from build123d import *

# Parameters (mm, degrees)
SKETCH_1_W          = 31
SKETCH_1_H          = 40
SKETCH_1_R          = 1.45
EXTRUDE_1_DEPTH     = 3
SKETCH_2_W          = 17
SKETCH_2_H          = 13
CUT_EXTRUDE_1_DEPTH = 3
FILLET_1_R          = 1.5


with BuildPart() as part:
    # 草图1 → 凸台-拉伸1 (new body)
    with BuildSketch(Plane.XY):
        with Locations((15.5, 20)):
            Rectangle(SKETCH_1_W, SKETCH_1_H)
        with Locations((4, 30)):
            Circle(SKETCH_1_R, mode=Mode.SUBTRACT)
        with Locations((4, 20)):
            Circle(SKETCH_1_R, mode=Mode.SUBTRACT)
        with Locations((4, 10)):
            Circle(SKETCH_1_R, mode=Mode.SUBTRACT)
        with Locations((27, 30)):
            Circle(SKETCH_1_R, mode=Mode.SUBTRACT)
        with Locations((27, 20)):
            Circle(SKETCH_1_R, mode=Mode.SUBTRACT)
        with Locations((27, 10)):
            Circle(SKETCH_1_R, mode=Mode.SUBTRACT)
    extrude(amount=EXTRUDE_1_DEPTH)

    # 草图2 → 切除-拉伸1 (cut)
    with BuildSketch(Plane.XY.offset(3)):
        with Locations((15.5, 28.5)):
            Rectangle(SKETCH_2_W, SKETCH_2_H)
        with Locations((15.5, 11.5)):
            Rectangle(SKETCH_2_W, SKETCH_2_H)
    extrude(amount=-CUT_EXTRUDE_1_DEPTH, mode=Mode.SUBTRACT)

    # 圆角1
    fillet_1_edges = [part.edges().sort_by_distance(p)[0] for p in [
        (7, 22, 1.5),
        (7, 35, 1.5),
        (24, 35, 1.5),
        (24, 22, 1.5),
        (7, 5, 1.5),
        (7, 18, 1.5),
        (24, 18, 1.5),
        (24, 5, 1.5),
        (0, 40, 1.5),
        (31, 40, 1.5),
        (31, 0, 1.5),
        (0, 0, 1.5),
    ]]
    fillet(fillet_1_edges, radius=FILLET_1_R)


solid = part.part
Geometry: final body of the model. Coordinates: model frame, mm. A direction names the side the tool comes from. Give positions to 0.01 mm unless a question says otherwise; leave off trailing zeros. Loops run counter-clockwise (first coordinate to the right, second up) from the corner with the lowest first, then second, coordinate; pieces in that order, holes last. Notation, with made-up numbers: M 34.25,-22.75 L 41.25,-22.75 A3 ccw 41.25,-17.75 Z; hole C -36.5,52.25 d6. An arc over 180 degrees is marked long. Put each result on its own line as item: value.
1) Cut plane B-B, the plane x = 9.5. Return the cut outline in (y, z), plus the area to 3 significant figures.
Computed values:
outline: M 0,0 L 5,0 L 5,3 L 0,3 Z; M 18,0 L 22,0 L 22,3 L 18,3 Z; M 35,0 L 40,0 L 40,3 L 35,3 Z
area: 42.0 mm^2
2) Mould query, pull axis X, two halves, no side actions, for faces 3 (the cylindrical face through (30.55, 39.57, 1.52)), 4 (the flat face through (15, 20, 0)), 5 (the cylindrical face through (28.339, 9.445, 1.479)). Classes: released by +X, released by -X, zero draft, split by the parting line, or undercut.
Computed values:
face 3: released by +X
face 4: zero draft
face 5: undercut
3) Reachability of faces 1 (the cylindrical face through (0.43, 39.55, 1.52)), 2 (the flat face through (7, 11, 2)) from +Z, -Z, +X, -X, +Y, -Y: full face, straight path, thin tool, end or side. Return the list, or none.
Computed values:
face 1: +Z, -Z, -X, +Y
face 2: +Z, -Z
4) Cut plane D-D, the plane y = 30. Return the cut outline in (x, z), plus the area to 3 significant figures.
Computed values:
outline: M 0,0 L 2.55,0 L 2.55,3 L 0,3 Z; M 5.45,0 L 7,0 L 7,3 L 5.45,3 Z; M 24,0 L 25.55,0 L 25.55,3 L 24,3 Z; M 28.45,0 L 31,0 L 31,3 L 28.45,3 Z
area: 24.6 mm^2
5) Cut plane C-C, the plane z = 2.15. Give the number of separate pieces and of enclosed holes in the cut face, plus the area to 3 significant figures.
Computed values:
separate pieces: 1
enclosed holes: 8
area: 760 mm^2
6) Cut plane A-A, the plane y = 7. Return the cut outline in (x, z), plus the area to 3 significant figures.
Computed values:
outline: M 0,0 L 7,0 L 7,3 L 0,3 Z; M 24,0 L 31,0 L 31,3 L 24,3 Z
area: 42.0 mm^2
7) Material intervals for L1, parallel to Y at x = 27, z = 0.9; L2, parallel to Y at x = 11, z = 0.3; L3, parallel to Y at x = 7.5, z = 2.5, sorted ascending. Write a range as from..to.
Computed values:
L1: y = 0..8.55, 11.45..18.55, 21.45..28.55, 31.45..40
L2: y = 0..5, 18..22, 35..40
L3: y = 0..5.38, 17.62..22.38, 34.62..40
